```python
from build123d import *

# Parameters (mm, degrees)
SKETCH1_W                                           = 50
SKETCH1_H                                           = 50
BOSS_EXTRUDE1_DEPTH                                 = 5
SKETCH3_W                                           = 37.499690969
SKETCH3_H                                           = 12.500309031
SKETCH3_W_2                                         = 12.500309031
SKETCH3_H_2                                         = 37.499690969
BOSS_EXTRUDE2_DEPTH                                 = 12
SKETCH5_W                                           = 37.499690969
SKETCH5_H                                           = 5
BOSS_EXTRUDE3_DEPTH                                 = 10
SKETCH6_W                                           = 27.499690969
SKETCH6_H                                           = 5
BOSS_EXTRUDE4_DEPTH                                 = 9
FILLET2_R                                           = 5
CBORE_FOR_3_BINDING_HEAD_MACHINE_SCREW1_D           = 2.794
CBORE_FOR_3_BINDING_HEAD_MACHINE_SCREW1_CBORE_D     = 5.95376
CBORE_FOR_3_BINDING_HEAD_MACHINE_SCREW1_CBORE_DEPTH = 1.4986


with BuildPart() as part:
    # Sketch1 → Boss-Extrude1 (new body)
    with BuildSketch(Plane(origin=(0, 0, 0), x_dir=(1, 0, 0), z_dir=(0, 1, 0))):
        Rectangle(SKETCH1_W, SKETCH1_H)
    extrude(amount=BOSS_EXTRUDE1_DEPTH)

    # Sketch3 → Boss-Extrude2 (add)
    with BuildSketch(Plane(origin=(0, 5, 0), x_dir=(1, 0, 0), z_dir=(0, 1, 0))):
        with Locations((-6.250154515, 18.749845484)):
            Rectangle(SKETCH3_W, SKETCH3_H)
        with Locations((18.749845484, 18.749845484)):
            Rectangle(SKETCH3_W_2, SKETCH3_H)
        with Locations((18.749845484, -6.250154515)):
            Rectangle(SKETCH3_W_2, SKETCH3_H_2)
    extrude(amount=BOSS_EXTRUDE2_DEPTH)

    # Sketch5 → Boss-Extrude3 (add)
    with BuildSketch(Plane.XY.offset(-12.499690969)):
        with Locations((-6.250154515, 14.5)):
            Rectangle(SKETCH5_W, SKETCH5_H)
    extrude(amount=BOSS_EXTRUDE3_DEPTH)

    # Sketch6 → Boss-Extrude4 (add)
    with BuildSketch(Plane.ZY.offset(-12.499690969)):
        with Locations((11.250154516, 14.5)):
            Rectangle(SKETCH6_W, SKETCH6_H)
    extrude(amount=BOSS_EXTRUDE4_DEPTH)

    # Fillet2
    fillet2_edges = [part.edges().sort_by_distance(p)[0] for p in [
        (0, 0, 25),
        (-25, 0, 0),
        (0, 0, -25),
        (25, 8.5, -25),
        (-25, 8.5, -25),
        (25, 17, 0),
        (0, 17, -25),
        (-25, 17, -13.749845484),
        (3.499690969, 17, 11.250154516),
        (-10.750154516, 17, -2.499690969),
        (14.249845484, 17, 25),
        (25, 8.5, 25),
        (25, 0, 0),
    ]]
    fillet(fillet2_edges, radius=FILLET2_R - 0.0001)  # a hair under: the kernel refuses the full size

    # CBORE for #3 Binding Head Machine Screw1 (through all)
    with Locations(Plane(origin=(0, 0, 0), x_dir=(-1, 0, 0), z_dir=(0, -1, 0))):
        with Locations((0, 0)):
            CounterBoreHole(CBORE_FOR_3_BINDING_HEAD_MACHINE_SCREW1_D / 2, CBORE_FOR_3_BINDING_HEAD_MACHINE_SCREW1_CBORE_D / 2, CBORE_FOR_3_BINDING_HEAD_MACHINE_SCREW1_CBORE_DEPTH)


solid = part.part
```
Read the model definition and answer for the solid it produces. Units are mm, in the model's axes. A direction names the side the tool comes from. Coordinates: 2 decimals unless noted, no trailing zeros. Write each loop counter-clockwise with the first axis right and the second up, starting at its lowest first coordinate (ties: lowest second). Pieces come first, ordered by that corner, then holes. Notation, with made-up numbers: (53, 68.5) -> (58, 68.5) arc R30 ccw to (58, 96.5) -> close; hole circle Ø3 at (-10, 9.5). An arc over 180 degrees is marked (long way). Return JSON: item names as keys, results as strings.
1. A cutting plane is placed at B-B (z = -16). Determine the outline of the cut face in (x, y), and give its area (3 significant figures).
Found:
{"outline": "(-25, 5) arc R5 ccw to (-20, 0) -> (20, 0) arc R5 ccw to (25, 5) -> (25, 12) arc R5 ccw to (20, 17) -> (-20, 17) arc R5 ccw to (-25, 12) -> close", "area": "829 mm2"}
2. Each of these flat-tipped pins is pushed along its axis until it touches: P1, Ø3.5, axis at x = 0, z = 0, coming from the -Y side; P2, Ø7.5, axis at x = -12.5, y = 9, coming from the +Z side; P3, Ø1.5, axis at y = 14, z = -11.5, coming from the +X side. Where does it stop, or does it pass through?
Found:
{"P1": "y = 1.5", "P2": "z = -2.5", "P3": "x = 24.84"}
3. Find the intervals of material crossed by line 1 along Y through (x, z) = (11, 0.5); line 2 along Y through (x, z) = (1, 6); line 3 along X through (y, z) = (7.25, 1), in increasing order. Write a range as from..to.
Found:
{"line 1": "0..5, 12..17", "line 2": "0..5", "line 3": "12.5..25"}
4. A tool of negligible diameter and unlimited length cuts with its end or side. For faces 1 (the face through (12.5, 8, 7)), 2 (the face through (-8.02, 15.5, -3.93)), 3 (the face through (-24, 15, -11)), from which of +Z, -Z, +X, -X, +Y, -Y can it reach the whole face along a straight path? Write none if from no direction.
Found:
{"face 1": "+Z, -X", "face 2": "+Z, -X, +Y", "face 3": "+Z, -Z, -X, +Y"}
5. Determine the mould class of faces 4 (the face through (7, 12, -2)), 5 (the face through (23, 9, 24)), 6 (the face through (-7, 8, -12.5)), 7 (the face through (23, 1, 0)) for opening direction Y: pulls with the +Y half, pulls with the -Y half, needs draft (parallel to the pull), parting line crosses it, or undercut.
Found:
{"face 4": "undercut", "face 5": "needs draft", "face 6": "undercut", "face 7": "pulls with the -Y half"}
